Geometry check sheet. Reference: drawing and pictorial views, mm from the part's lowest x, y, z. A direction names the side the tool comes from. Coordinates: 2 decimals unless noted, no trailing zeros. Write each loop counter-clockwise with the first axis right and the second up, starting at its lowest first coordinate (ties: lowest second). Pieces come first, ordered by that corner, then holes. Notation, with made-up numbers: (38.5, 46) -> (93.5, 46) arc R8 ccw to (93.5, 52) -> close; hole circle Ø8 at (-11.75, -17.5). An arc over 180 degrees is marked (long way). Answer in a Markdown table with one row per item.
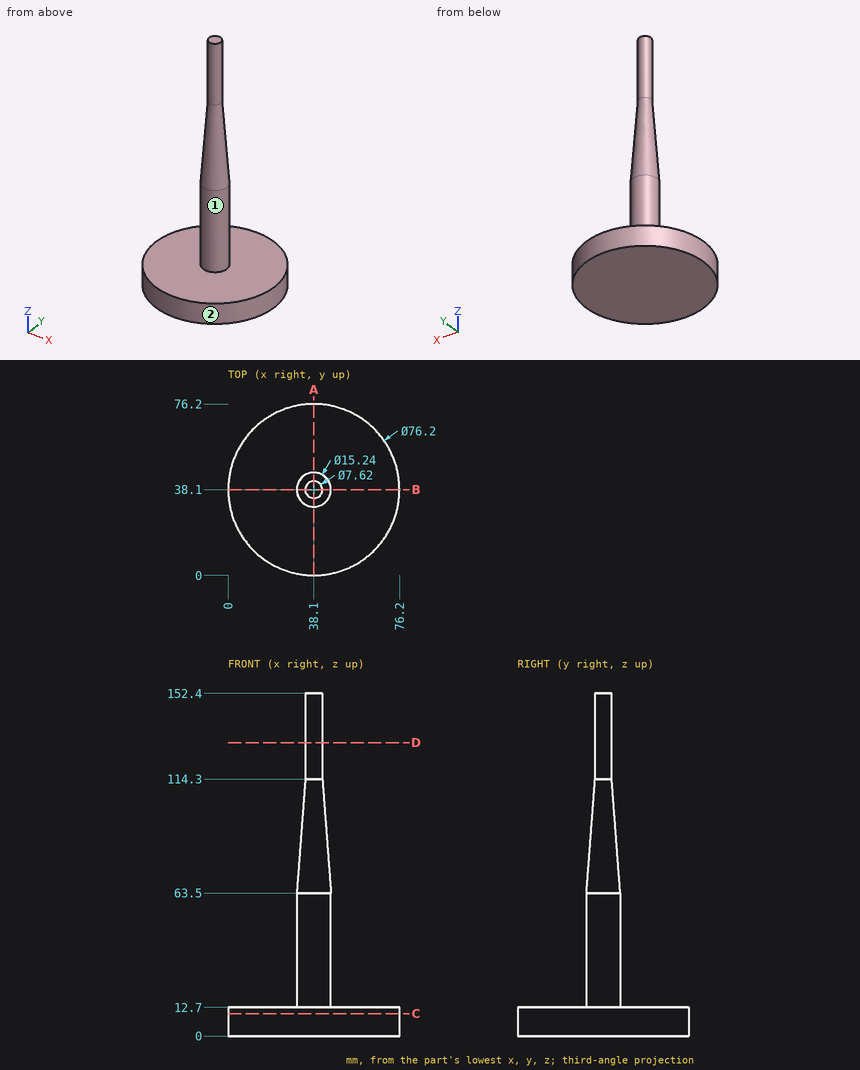
1. Section check C-C, the plane z = 10. Record the boundary of the cut face in (x, y).
Geometry says:
| item | result |
|---|---|
| outline | circle Ø76.2 at (38.1, 38.1) |
2. Depth check by flat-ended pin: P1, Ø2, axis at x = 39, y = 28, coming from the -Z side; P2, Ø12, axis at x = 65, y = 58.5, coming from the +Z side; P3, Ø3, axis at x = 39, z = 30.5, coming from the -Y side. Enter the tip coordinate at first touch or a pass-through.
Geometry says:
| item | result |
|---|---|
| P1 | z = 0 |
| P2 | z = 12.7 |
| P3 | y = 30.48 |
3. Thickness scan on line 1 (Z direction, x = 56.5, y = 6); line 2 (X direction, y = 42.5, z = 70); line 3 (Y direction, x = 39, z = 121). Record the ranges inside material, lowest first. Write a range as from..to.
Geometry says:
| item | result |
|---|---|
| line 1 | 0..12.7 |
| line 2 | 32.49..43.71 |
| line 3 | 34.4..41.8 |
4. Section check A-A, the plane x = 38.1. Record the boundary of the cut face in (y, z).
Geometry says:
| item | result |
|---|---|
| outline | (0, 0) -> (76.2, 0) -> (76.2, 12.7) -> (45.72, 12.7) -> (45.72, 63.5) -> (41.91, 114.3) -> (41.91, 152.4) -> (34.29, 152.4) -> (34.29, 114.3) -> (30.48, 63.5) -> (30.48, 12.7) -> (0, 12.7) -> close |
5. Section check D-D, the plane z = 130.5. Record the boundary of the cut face in (x, y), plus the area to 3 significant figures.
Geometry says:
| item | result |
|---|---|
| outline | circle Ø7.62 at (38.1, 38.1) |
| area | 45.6 mm^2 |
6. Tool access check on the marked faces 1 and 2. Record the directions out of +Z, -Z, +X, -X, +Y, -Y that give a thin tool (end or side, any length) a straight path to the whole face; none if there is none.
Geometry says:
| item | result |
|---|---|
| face 1 | +Z |
| face 2 | +Z, -Z |
